from build123d import *

# Parameters (mm, degrees)
SKETCH1_W                     = 47
SKETCH1_H                     = 27
BOSS_EXTRUDE1_DEPTH           = 3
SKETCH2_R                     = 2
BOSS_EXTRUDE2_DEPTH           = 7
BOSS_EXTRUDE2_DRAFT           = 5
BOSS_EXTRUDE2_PROFILE_2_DEPTH = 7
BOSS_EXTRUDE2_PROFILE_2_DRAFT = 5
BOSS_EXTRUDE2_PROFILE_3_DEPTH = 7
BOSS_EXTRUDE2_PROFILE_3_DRAFT = 5
BOSS_EXTRUDE2_PROFILE_4_DEPTH = 7
BOSS_EXTRUDE2_PROFILE_4_DRAFT = 5
SKETCH3_R                     = 2
CUT_EXTRUDE1_DEPTH            = 5


with BuildPart() as part:
    # Sketch1 → Boss-Extrude1 (new body)
    with BuildSketch(Plane.XY):
        Rectangle(SKETCH1_W, SKETCH1_H)
    extrude(amount=BOSS_EXTRUDE1_DEPTH)


with BuildPart() as boss_extrude2_tool:
    # Sketch2 → Boss-Extrude2 (with draft: the straight prism first)
    with BuildSketch(Plane(origin=(0, 0, 0), x_dir=(-1, 0, 0), z_dir=(0, 0, -1))):
        with Locations((-20, 10)):
            Circle(SKETCH2_R)
    extrude(amount=BOSS_EXTRUDE2_DEPTH)
    # Boss-Extrude2: the draft: its side faces are tilted about the plane it starts from
    boss_extrude2_sides = [boss_extrude2_tool.faces().sort_by_distance(p)[0] for p in [
        (22, 10, -3.5),
    ]]
    draft(boss_extrude2_sides, Plane(origin=(0, 0, 0), x_dir=(-1, 0, 0), z_dir=(0, 0, -1)), BOSS_EXTRUDE2_DRAFT)


with BuildPart() as part_1:
    add(part.part)

    # Boss-Extrude2: add boss_extrude2_tool
    add(boss_extrude2_tool.part)


with BuildPart() as boss_extrude2_profile_2_tool:
    # Sketch2 → Boss-Extrude2 profile 2 (with draft: the straight prism first)
    with BuildSketch(Plane(origin=(0, 0, 0), x_dir=(-1, 0, 0), z_dir=(0, 0, -1))):
        with Locations((20, 10)):
            Circle(SKETCH2_R)
    extrude(amount=BOSS_EXTRUDE2_PROFILE_2_DEPTH)
    # Boss-Extrude2 profile 2: the draft: its side faces are tilted about the plane it starts from
    boss_extrude2_profile_2_sides = [boss_extrude2_profile_2_tool.faces().sort_by_distance(p)[0] for p in [
        (-18, 10, -3.5),
    ]]
    draft(boss_extrude2_profile_2_sides, Plane(origin=(0, 0, 0), x_dir=(-1, 0, 0), z_dir=(0, 0, -1)), BOSS_EXTRUDE2_PROFILE_2_DRAFT)


with BuildPart() as part_2:
    add(part_1.part)

    # Boss-Extrude2 profile 2: add boss_extrude2_profile_2_tool
    add(boss_extrude2_profile_2_tool.part)


with BuildPart() as boss_extrude2_profile_3_tool:
    # Sketch2 → Boss-Extrude2 profile 3 (with draft: the straight prism first)
    with BuildSketch(Plane(origin=(0, 0, 0), x_dir=(-1, 0, 0), z_dir=(0, 0, -1))):
        with Locations((20, -10)):
            Circle(SKETCH2_R)
    extrude(amount=BOSS_EXTRUDE2_PROFILE_3_DEPTH)
    # Boss-Extrude2 profile 3: the draft: its side faces are tilted about the plane it starts from
    boss_extrude2_profile_3_sides = [boss_extrude2_profile_3_tool.faces().sort_by_distance(p)[0] for p in [
        (-18, -10, -3.5),
    ]]
    draft(boss_extrude2_profile_3_sides, Plane(origin=(0, 0, 0), x_dir=(-1, 0, 0), z_dir=(0, 0, -1)), BOSS_EXTRUDE2_PROFILE_3_DRAFT)


with BuildPart() as part_3:
    add(part_2.part)

    # Boss-Extrude2 profile 3: add boss_extrude2_profile_3_tool
    add(boss_extrude2_profile_3_tool.part)


with BuildPart() as boss_extrude2_profile_4_tool:
    # Sketch2 → Boss-Extrude2 profile 4 (with draft: the straight prism first)
    with BuildSketch(Plane(origin=(0, 0, 0), x_dir=(-1, 0, 0), z_dir=(0, 0, -1))):
        with Locations((-20, -10)):
            Circle(SKETCH2_R)
    extrude(amount=BOSS_EXTRUDE2_PROFILE_4_DEPTH)
    # Boss-Extrude2 profile 4: the draft: its side faces are tilted about the plane it starts from
    boss_extrude2_profile_4_sides = [boss_extrude2_profile_4_tool.faces().sort_by_distance(p)[0] for p in [
        (22, -10, -3.5),
    ]]
    draft(boss_extrude2_profile_4_sides, Plane(origin=(0, 0, 0), x_dir=(-1, 0, 0), z_dir=(0, 0, -1)), BOSS_EXTRUDE2_PROFILE_4_DRAFT)


with BuildPart() as part_4:
    add(part_3.part)

    # Boss-Extrude2 profile 4: add boss_extrude2_profile_4_tool
    add(boss_extrude2_profile_4_tool.part)

    # Sketch3 → Cut-Extrude1 (cut)
    with BuildSketch(Plane.XY.offset(3)):
        with Locations((5, 7.5)):
            Circle(SKETCH3_R)
        with Locations((5, -7.5)):
            Circle(SKETCH3_R)
    extrude(amount=-CUT_EXTRUDE1_DEPTH, mode=Mode.SUBTRACT)


solid = part_4.part
Source: CAD feature listing. Evaluate the final solid. Frame: model axes, mm. A direction names the side the tool comes from. Round coordinates to 2 decimals unless told otherwise and drop trailing zeros. Loops run counter-clockwise (first coordinate to the right, second up) from the corner with the lowest first, then second, coordinate; pieces in that order, holes last. Notation, with made-up numbers: (19, 29) - (47, 29) arc R34 cw to (47, 65) - close; hole circle Ø9 at (11, 21.25). An arc over 180 degrees is marked (long way). Write item = value, one per line. Start each with the question number.
Item 1: Section query D-D on x = -20. Output: boundary loops of the cut face in (y, z), plus the area to 3 significant figures.
Item 2: Section query A-A on y = 7.5. Output: boundary loops of the cut face in (x, z), plus the area to 3 significant figures.
Item 3: Mould query, pull axis Y, two halves, no side actions, for faces 3 (the face through (0, 13.5, 1)), 4 (the face through (20, 10, -7)), 5 (the face through (3.002, -7.412, 1.521)). Classes: released by +Y, released by -Y, zero draft, split by the parting line, or undercut.
Item 4: First-contact query: pin 1 Ø10 at (x, y) = (-8.5, -8.5) entering from -Z; pin 2 Ø2 at (y, z) = (9.5, -3.5) entering from -X; pin 3 Ø6.5 at (x, y) = (5, 7.5) entering from +Z. Flat tips, straight axial feed; report the tip coordinate or a pass-through.
Item 5: Reachability of faces 1 (the face through (0, 0, 0)), 2 (the face through (3.526, 8.852, 1.521)) from +Z, -Z, +X, -X, +Y, -Y: full face, straight path, thin tool, end or side. Return the list, or none.
Item 6: Section query C-C on z = 0.5. Output: boundary loops of the cut face in (x, y).
Item 7: Material intervals for line 1 (Y direction, x = 5, z = 0.8); line 2 (X direction, y = -10.5, z = -5.5); line 3 (Z direction, x = 2.5, y = -7.25), sorted ascending.
Item 8: Section query B-B on x = 5. Output: boundary loops of the cut face in (y, z).
Results list:
q1.outline = (-13.5, 0) - (-12, 0) - (-11.39, -7) - (-8.61, -7) - (-8, 0) - (8, 0) - (8.61, -7) - (11.39, -7) - (12, 0) - (13.5, 0) - (13.5, 3) - (-13.5, 3) - close
q1.area = 128 mm²
q2.outline = (-23.5, 0) - (3, 0) - (3, 3) - (-23.5, 3) - close; (7, 0) - (23.5, 0) - (23.5, 3) - (7, 3) - close
q2.area = 129 mm²
q3.face_3 = released by +Y
q3.face_4 = zero draft
q3.face_5 = undercut
q4.pin_1 = 0
q4.pin_2 = -21.77
q4.pin_3 = 3
q5.face_1 = -Z
q5.face_2 = +Z, -Z
q6.outline = (-23.5, -13.5) - (23.5, -13.5) - (23.5, 13.5) - (-23.5, 13.5) - close; hole circle Ø4 at (5, -7.5); hole circle Ø4 at (5, 7.5)
q7.line_1 = -13.5 to -9.5, -5.5 to 5.5, 9.5 to 13.5
q7.line_2 = -21.43 to -18.57, 18.57 to 21.43
q7.line_3 = 0 to 3
q8.outline = (-13.5, 0) - (-9.5, 0) - (-9.5, 3) - (-13.5, 3) - close; (-5.5, 0) - (5.5, 0) - (5.5, 3) - (-5.5, 3) - close; (9.5, 0) - (13.5, 0) - (13.5, 3) - (9.5, 3) - close
